Input: part model. Units: mm. Frame: model coordinates. Face numbers are marked on the shaded views. A direction names the side the tool comes from. Give positions to 0.01 mm unless a question says otherwise; leave off trailing zeros. Loops run counter-clockwise (first coordinate to the right, second up) from the corner with the lowest first, then second, coordinate; pieces in that order, holes last. Notation, with made-up numbers: (57, 35) -> (85, 35) arc R14 ccw to (85, 44) -> close; hole circle Ø11 at (4, 83.25). An arc over 180 degrees is marked (long way). Answer in a Markdown table with one row per item. Add a question column.
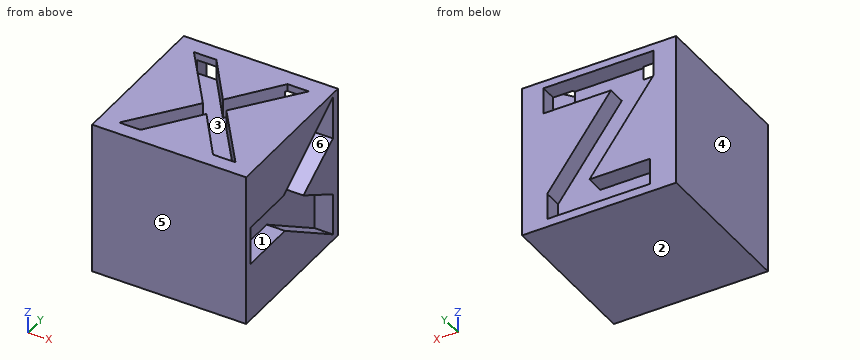
Autodesk Inventor part; units mm, degrees
ref_plane "YZ Plane" through (0, 0, 0) normal (1, 0, 0) x (0, 1, 0)
ref_plane "XZ Plane" through (0, 0, 0) normal (0, 1, 0) x (-1, 0, 0)
ref_plane "XY Plane" through (0, 0, 0) normal (0, 0, 1) x (1, 0, 0)
sketch "Sketch3" plane through (0, 0, 0) normal (0, 0, 1) x (1, 0, 0)
  line L0 (12.7, -12.7) -> (-12.7, -12.7)
  line L1 (-12.7, -12.7) -> (-12.7, 12.7)
  line L2 (-12.7, 12.7) -> (12.7, 12.7)
  line L3 (12.7, 12.7) -> (12.7, -12.7)
  line L4 (12.7, -12.7) -> (-12.7, 12.7) construction
  line L5 (-12.7, -12.7) -> (12.7, 12.7) construction
  point P0 (0, 0)
  dimension "d0" = 25.4
  dimension "d1" = 25.4
extrude "Cubo" add sketch "Sketch3" along normal blind 25.4
sketch "Sketch5" plane through (0, 0, 25.4) normal (0, 0, 1) x (1, 0, 0)
  line L0 (-12.1868, 12.0555) -> (12.0292, 12.0555) construction
  line L1 (12.0292, 12.0555) -> (12.0292, -12.3181) construction
  line L2 (12.0292, -12.3181) -> (-12.1868, -12.3181) construction
  line L3 (-12.1868, -12.3181) -> (-12.1868, 12.0555) construction
  line L4 (9.4966, -10.2913) -> (5.7916, -10.2913)
  line L5 (5.7916, -10.2913) -> (-0.1365, -2.1567)
  line L6 (-0.1365, -2.1567) -> (-6.1633, -10.2913)
  line L7 (-6.1633, -10.2913) -> (-9.6707, -10.2913)
  line L8 (-9.6707, -10.2913) -> (-1.9149, -0.1313)
  line L9 (-1.9149, -0.1313) -> (-9.4402, 10.0287)
  line L10 (-9.4402, 10.0287) -> (-5.7352, 10.0287)
  line L11 (-5.7352, 10.0287) -> (0.0776, 2.0588)
  line L12 (0.0776, 2.0588) -> (5.9892, 10.0287)
  line L13 (5.9892, 10.0287) -> (9.4966, 10.0287)
  line L14 (9.4966, 10.0287) -> (1.856, 0.0169)
  line L15 (1.856, 0.0169) -> (9.4966, -10.2913)
  point P0 (0, 0)
extrude "X" cut sketch "Sketch5" against normal blind 3.175
sketch "Esboço9" plane through (12.7, -12.7, 0) normal (1, 0, 0) x (0, 0, -1)
  line L0 (-24.9757, 24.9816) -> (-0.1587, 24.9816) construction
  line L1 (-0.1587, 24.9816) -> (-0.1587, 0.228) construction
  line L2 (-0.1587, 0.228) -> (-24.9757, 0.228) construction
  line L3 (-24.9757, 0.228) -> (-24.9757, 24.9816) construction
  line L4 (-0.989, 24.0348) -> (-9.6587, 10.7152)
  line L5 (-9.6587, 10.7152) -> (-9.6587, 1.1748)
  line L6 (-9.6587, 1.1748) -> (-15.9573, 1.1748)
  line L7 (-15.9573, 1.1748) -> (-15.9573, 10.4374)
  line L8 (-15.9573, 10.4374) -> (-24.7752, 24.0348)
  line L9 (-24.7752, 24.0348) -> (-17.606, 24.0348)
  line L10 (-17.606, 24.0348) -> (-12.6783, 15.8652)
  line L11 (-12.6783, 15.8652) -> (-7.9359, 24.0348)
  line L12 (-7.9359, 24.0348) -> (-0.989, 24.0348)
  point P0 (0, 12.7)
extrude "Extrusão6" cut sketch "Esboço9" against normal blind 3
sketch "Esboço10" plane through (-12.7, 12.7, 0) normal (0, 1, 0) x (1, 0, 0)
  line L0 (0.3012, -0.2854) -> (25.0988, -0.2854) construction
  line L1 (25.0988, -0.2854) -> (25.0988, -25.2732) construction
  line L2 (25.0988, -25.2732) -> (0.3012, -25.2732) construction
  line L3 (0.3012, -25.2732) -> (0.3012, -0.2854) construction
  line L4 (21.8699, -24.2093) -> (3.7524, -24.2093)
  line L5 (3.7524, -24.2093) -> (3.7524, -19.93)
  line L6 (3.7524, -19.93) -> (14.2932, -5.7027)
  line L7 (14.2932, -5.7027) -> (4.3081, -5.7027)
  line L8 (4.3081, -5.7027) -> (4.3081, -1.3493)
  line L9 (4.3081, -1.3493) -> (21.2586, -1.3493)
  line L10 (21.2586, -1.3493) -> (21.2586, -5.7027)
  line L11 (21.2586, -5.7027) -> (10.7549, -19.8559)
  line L12 (10.7549, -19.8559) -> (21.8699, -19.8559)
  line L13 (21.8699, -19.8559) -> (21.8699, -24.2093)
  point P0 (12.7, 0)
extrude "Extrusão7" cut sketch "Esboço10" against normal blind 3
properties part number "Cubo_3DPrint"
1) Pin query (flat end, axial travel): pin 1 (6 mm diameter, centred on x = -2.5, y = -3, fed in from +Z). Return the tip coordinate at first contact, or that it passes through.
2) Material intervals for line 1 along X through (y, z) = (-3.5, 24.25); line 2 along Z through (x, y) = (-7.25, -7.75) (3 decimals); line 3 along X through (y, z) = (9.75, 20.75), sorted ascending.
3) Section A-A on x = 11. Output: boundary loops of the cut face in (y, z).
4) Section C-C on y = 9. Output: boundary loops of the cut face in (x, z) (3 decimals).
5) Section D-D on z = 13.5. Output: boundary loops of the cut face in (x, y), and give its area (3 significant figures).
6) Section B-B on z = 23.75. Output: boundary loops of the cut face in (x, y).
7) Reachability of the marked faces 1, 2 and 3 from +Z, -Z, +X, -X, +Y, -Y: full face, straight path, thin tool, end or side. Return the list, or none.
8) Pull-direction query (Y, two-part tool) for the marked faces 4, 5 and 6; classes: +Y half, -Y half, draft (parallel to the pull), parting line (faces both ways), or undercut.
Working result:
| question | item | result |
|---|---|---|
| 1 | pin 1 | stops at z = 25.4 |
| 2 | line 1 | x = -12.7 to -4.49, -1.13 to 0.84, 4.46 to 12.7 |
| 2 | line 2 | z = 0 to 22.225 |
| 2 | line 3 | x = -12.7 to -8.95, 9.17 to 9.7 |
| 3 | outline | (-12.7, 0) -> (12.7, 0) -> (12.7, 25.4) -> (-12.7, 25.4) -> close; hole (-11.53, 9.66) -> (-1.98, 9.66) -> (11.33, 0.99) -> (11.33, 7.94) -> (3.17, 12.68) -> (11.33, 17.61) -> (11.33, 24.78) -> (-2.26, 15.96) -> (-11.53, 15.96) -> close |
| 4 | outline | (-12.7, 0) -> (12.7, 0) -> (12.7, 2.509) -> (9.7, 2.509) -> (9.7, 9.291) -> (12.7, 9.291) -> (12.7, 16.198) -> (9.7, 16.198) -> (9.7, 23.261) -> (12.7, 23.261) -> (12.7, 25.4) -> (8.712, 25.4) -> (8.712, 22.225) -> (5.226, 22.225) -> (5.226, 25.4) -> (-4.985, 25.4) -> (-4.985, 22.225) -> (-8.678, 22.225) -> (-8.678, 25.4) -> (-12.7, 25.4) -> close |
| 5 | outline | (-12.7, -12.7) -> (12.7, -12.7) -> (12.7, -11.53) -> (9.7, -11.53) -> (9.7, 4.53) -> (12.7, 4.53) -> (12.7, 12.7) -> (2.77, 12.7) -> (2.77, 9.7) -> (-4.18, 9.7) -> (-4.18, 12.7) -> (-12.7, 12.7) -> close |
| 5 | area | 576 mm2 |
| 6 | outline | (-12.7, -12.7) -> (12.7, -12.7) -> (12.7, 9.75) -> (9.7, 9.75) -> (9.7, 11.33) -> (12.7, 11.33) -> (12.7, 12.7) -> (9.17, 12.7) -> (9.17, 10.03) -> (9.5, 10.03) -> (1.86, 0.02) -> (9.5, -10.29) -> (5.79, -10.29) -> (-0.14, -2.16) -> (-6.16, -10.29) -> (-9.67, -10.29) -> (-1.91, -0.13) -> (-9.44, 10.03) -> (-8.95, 10.03) -> (-8.95, 12.7) -> (-12.7, 12.7) -> close; (-5.5, 9.7) -> (0.08, 2.06) -> (5.75, 9.7) -> close |
| 7 | face 1 | +X |
| 7 | face 2 | -Z, +X, -X, +Y, -Y |
| 7 | face 3 | +Z |
| 8 | face 4 | draft |
| 8 | face 5 | -Y half |
| 8 | face 6 | undercut |
